Design review of the part built by this model. Coordinates are the model's own, in mm. Face numbers are marked on the shaded views. A direction names the side the tool comes from. Coordinates: 2 decimals unless noted, no trailing zeros. Loops run counter-clockwise (first coordinate to the right, second up) from the corner with the lowest first, then second, coordinate; pieces in that order, holes last. Notation, with made-up numbers: (14, 25) - (73, 25) arc R30 ccw to (73, 53) - close; hole circle Ø11 at (-31.75, 24). An arc over 180 degrees is marked (long way). Return JSON: item names as keys, results as strings. Group by question number.
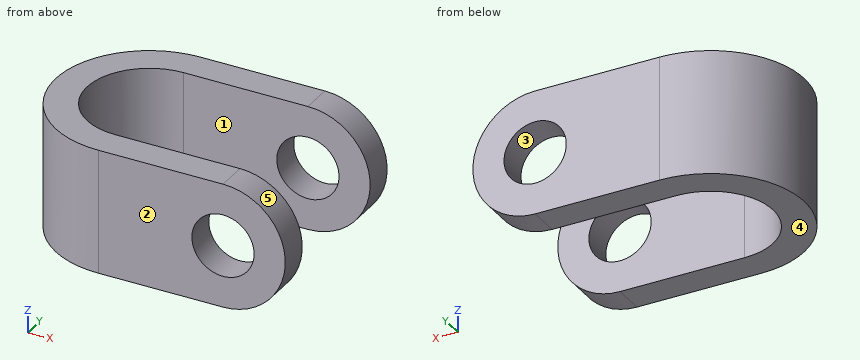
from build123d import *

# Parameters (mm, degrees)
EXTRUDE_THIN1_DEPTH = 90
SKETCH2_R           = 10
BOSS_EXTRUDE1_DEPTH = 90


with BuildPart() as part:
    # Sketch1 → Extrude-Thin1 (new body)
    with BuildSketch(Plane.XY):
        with BuildLine():
            Line((0, -15), (-60, -15))
            ThreePointArc((-60, -15), (-80, -35), (-60, -55))
            Line((-60, -55), (0, -55))
            Line((0, -55), (0, -65))
            Line((0, -65), (-60, -65))
            ThreePointArc((-60, -65), (-90, -35), (-60, -5))
            Line((-60, -5), (0, -5))
            Line((0, -5), (0, -15))
        make_face()
    extrude(amount=EXTRUDE_THIN1_DEPTH)


with BuildPart() as body_2:
    # Sketch2 → Boss-Extrude1 (new body)
    with BuildSketch(Plane(origin=(0, 0, 0), x_dir=(1, 0, 0), z_dir=(0, 1, 0))):
        with BuildLine():
            Line((-90, -25), (-90, -65))
            Line((-90, -65), (-20, -65))
            ThreePointArc((-20, -65), (0, -45), (-20, -25))
            Line((-20, -25), (-90, -25))
        make_face()
        with Locations(Location((-20, -45, 0), (0, 0, 270))):
            Circle(SKETCH2_R, mode=Mode.SUBTRACT)
    extrude(amount=-BOSS_EXTRUDE1_DEPTH)

    # Combine1: intersect part
    add(part.part, mode=Mode.INTERSECT)


solid = body_2.part
Item 1: Add section D-D (y = -35). State the section outline as (x, z) points, then the cut area to 3 significant figures.
Item 2: Add section A-A (z = 45). State the section outline as (x, y) points, then the cut area to 3 significant figures.
Item 3: For the marked faces 1 and 2, list the 3-axis set-ups (+Z, -Z, +X, -X, +Y, -Y) from which the entire face can be reached by the end or side of a thin tool; tool diameter is ignored.
Item 4: To check wall thickness, follow line 1 (Y direction, x = -54.5, z = 27); line 2 (X direction, y = -61.5, z = 45); line 3 (X direction, y = -57, z = 45.5). State the ranges of each line that lie inside material, in increasing order. Write a range as from..to.
Item 5: Draft analysis for pull direction X (two halves, no side actions). For the marked faces 3, 4 and 5, state which applies: pulls with the +X half, pulls with the -X half, needs draft (parallel to the pull), parting line crosses it, or undercut.
Item 6: For P1, Ø12, axis at y = -36.5, z = 58, coming from the -X side; P2, Ø3, axis at x = -76, z = 55.5, coming from the -Y side; P3, Ø10, axis at x = -76.5, z = 50.5, coming from the +Y side, all flat-tipped, find the tip position at first contact; note any pin that passes through.
Item 7: Add section B-B (x = -50). State the section outline as (y, z) points, then the cut area to 3 significant figures.
Item 8: Add section C-C (z = 28). State the section outline as (x, y) points, then the cut area to 3 significant figures.
Answers below:
{
 "1": {"outline": "(-90, 25) - (-80, 25) - (-80, 65) - (-90, 65) - close", "area": "400 mm^2"},
 "2": {"outline": "(-60, -65) - (-30, -65) - (-30, -55) - (-60, -55) arc R20 cw to (-60, -15) - (-30, -15) - (-30, -5) - (-60, -5) arc R30 ccw to start; (-10, -65) - (0, -65) - (0, -55) - (-10, -55) - close; (-10, -15) - (0, -15) - (0, -5) - (-10, -5) - close", "area": "1,590 mm^2"},
 "3": {"face 1": "+Z, -Z, +X", "face 2": "+Z, -Z, +X, -X, -Y"},
 "4": {"line 1": "y = -65..-55, -15..-5", "line 2": "x = -74.06..-30, -10..0", "line 3": "x = -80.4..-29.99, -10.01..-0.01"},
 "5": {"face 3": "undercut", "face 4": "needs draft", "face 5": "pulls with the +X half"},
 "6": {"P1": "stops at x = -90", "P2": "stops at y = -61.26", "P3": "stops at y = -7.29"},
 "7": {"outline": "(-65, 25) - (-55, 25) - (-55, 65) - (-65, 65) - close; (-15, 25) - (-5, 25) - (-5, 65) - (-15, 65) - close", "area": "800 mm^2"},
 "8": {"outline": "(-60, -65) - (-9.46, -65) - (-9.46, -55) - (-60, -55) arc R20 cw to (-60, -15) - (-9.46, -15) - (-9.46, -5) - (-60, -5) arc R30 ccw to start", "area": "1,800 mm^2"}
}
